For this review, take the finished solid that the model builds, in its own axes (mm). A direction names the side the tool comes from. Round coordinates to 2 decimals unless told otherwise and drop trailing zeros. Order: outer loops, then holes, each group sorted by start corner. A loop starts at its lowest first (then second) coordinate and runs counter-clockwise, first axis right, second up. Notation, with made-up numbers: (2.5, 55) - (40.5, 55) arc R16 ccw to (40.5, 60) - close; hole circle Ø7 at (65.5, -18.75). An arc over 180 degrees is marked (long way). One line per question, with ' | ' between items.
```python
from build123d import *

# Parameters (mm, degrees)
SKETCH1_W           = 5.75
SKETCH1_H           = 15.43
BOSS_EXTRUDE3_DEPTH = 11
SKETCH3_R           = 1
BOSS_EXTRUDE4_DEPTH = 3.086
SKETCH4_R           = 1
BOSS_EXTRUDE5_DEPTH = 1.543
BOSS_EXTRUDE6_START = -3.086
SKETCH5_R           = 1
BOSS_EXTRUDE6_DEPTH = 3.086


with BuildPart() as part:
    # Sketch1 → Boss-Extrude3 (new body)
    with BuildSketch(Plane(origin=(0, 0, 0), x_dir=(1, 0, 0), z_dir=(0, 1, 0))):
        with Locations((21.975, 0)):
            Rectangle(SKETCH1_W, SKETCH1_H)
    extrude(amount=BOSS_EXTRUDE3_DEPTH)

    # Sketch3 → Boss-Extrude4 (add)
    with BuildSketch(Plane(origin=(0, 0, -7.715), x_dir=(-1, 0, 0), z_dir=(0, 0, -1))):
        with BuildLine():
            Line((-24.85, 11), (-24.85, 6.250173181))
            Line((-24.85, 6.250173181), (-27.653680617, 6.250173181))
            ThreePointArc((-27.653680617, 6.250173181), (-29.999956704, 8.63934057), (-27.625, 11))
            Line((-27.625, 11), (-24.85, 11))
        make_face()
        with Locations((-27.625, 8.625)):
            Circle(SKETCH3_R, mode=Mode.SUBTRACT)
    extrude(amount=-BOSS_EXTRUDE4_DEPTH)

    # Sketch4 → Boss-Extrude5 (add, symmetric)
    with BuildSketch(Plane.XY):
        with BuildLine():
            Line((27.625, 11), (24.85, 11))
            Line((24.85, 11), (24.85, 6.250173181))
            Line((24.85, 6.250173181), (27.653680617, 6.250173181))
            ThreePointArc((27.653680617, 6.250173181), (29.999956704, 8.63934057), (27.625, 11))
        make_face()
        with Locations(Location((27.625, 8.625, 0), (0, 0, 180))):
            Circle(SKETCH4_R, mode=Mode.SUBTRACT)
    extrude(amount=BOSS_EXTRUDE5_DEPTH, both=True)

    # Sketch5 → Boss-Extrude6 (add)
    with BuildSketch(Plane.XY.offset(7.715).offset(BOSS_EXTRUDE6_START)):
        with BuildLine():
            Line((24.85, 6.250173181), (27.653680617, 6.250173181))
            ThreePointArc((27.653680617, 6.250173181), (29.999956704, 8.63934057), (27.625, 11))
            Line((27.625, 11), (24.85, 11))
            Line((24.85, 11), (24.85, 6.250173181))
        make_face()
        with Locations(Location((27.625, 8.625, 0), (0, 0, 180))):
            Circle(SKETCH5_R, mode=Mode.SUBTRACT)
    extrude(amount=BOSS_EXTRUDE6_DEPTH)


solid = part.part
```
(1) For probe 1 along Z at (x, y) = (25.25, 6.75) (3 decimals); probe 2 along X at (y, z) = (0.5, 4.75); probe 3 along Y at (x, z) = (25.5, 1.5), list the stretches that pass through material, from the lowest coordinate up. Write a range as [from, to].
Output values:
probe 1: [-7.715, -4.629], [-1.543, 1.543], [4.629, 7.715] | probe 2: [19.1, 24.85] | probe 3: [6.25, 11]
(2) We need section D-D on x = 29. State the section outline as (y, z) points (1 decimal), plus the area to 3 significant figures.
Output values:
outline: (6.7, -7.7) - (10.6, -7.7) - (10.6, -4.6) - (6.7, -4.6) - close; (6.7, -1.5) - (10.6, -1.5) - (10.6, 1.5) - (6.7, 1.5) - close; (6.7, 4.6) - (10.6, 4.6) - (10.6, 7.7) - (6.7, 7.7) - close | area: 35.9 mm^2
(3) For faces 5 (the flat face through (24.85, 4, 0)), 6 (the cylindrical face through (27.755, 7.634, -0.022)), 7 (the flat face through (26, 6.25, 6)), 8 (the flat face through (26, 9, 1.543)), list the 3-axis set-ups (+Z, -Z, +X, -X, +Y, -Y) from which the entire face can be reached by the end or side of a thin tool; tool diameter is ignored.
Output values:
face 5: +X, -Y | face 6: +Z, -Z | face 7: +Z, -Z, +X, -Y | face 8: +X, +Y, -Y
(4) We need section B-B on z = 5. State the section outline as (x, y) points (3 decimals), plus the area to 3 significant figures.
Output values:
outline: (19.1, 0) - (24.85, 0) - (24.85, 6.25) - (27.654, 6.25) arc R2.375 ccw to (27.625, 11) - (19.1, 11) - close; hole circle Ø2 at (27.625, 8.625) | area: 82.1 mm^2
(5) Insertion check: pin 1 (1.4 mm diameter, centred on x = 27, z = 6.5, fed in from -Y); pin 2 (1.5 mm diameter, centred on y = 7.5, z = -6, fed in from +X); pin 3 (1.5 mm diameter, centred on x = 27.5, y = 1.5, fed in from -Z) (3 decimals); pin 4 (4 mm diameter, centred on y = 5.5, z = 5.5, fed in from +X). Each pin has a flat end and moves straight along its axis. Give the tip position at first contact, or say it passes through.
Output values:
pin 1: y = 6.25 | pin 2: x = 29.97 | pin 3: through | pin 4: x = 29.72
(6) We need section A-A on x = 27.25. State the section outline as (y, z) points (3 decimals), plus the area to 3 significant figures.
Output values:
outline: (6.25, -7.715) - (7.698, -7.715) - (7.698, -4.629) - (6.25, -4.629) - close; (6.25, -1.543) - (7.698, -1.543) - (7.698, 1.543) - (6.25, 1.543) - close; (6.25, 4.629) - (7.698, 4.629) - (7.698, 7.715) - (6.25, 7.715) - close; (9.552, -7.715) - (11, -7.715) - (11, -4.629) - (9.552, -4.629) - close; (9.552, -1.543) - (11, -1.543) - (11, 1.543) - (9.552, 1.543) - close; (9.552, 4.629) - (11, 4.629) - (11, 7.715) - (9.552, 7.715) - close | area: 26.8 mm^2
(7) Mouldability with a two-part tool opening along Z and no side actions: class faces 1 (the flat face through (26, 9, -1.543)), 2 (the cylindrical face through (27.755, 9.616, -6.194)), 3 (the flat face through (23, 6, -7.715)), 4 (the flat face through (26, 9, 4.629)) as released by +Z, released by -Z, zero draft, split by the parting line, or undercut.
Output values:
face 1: undercut | face 2: zero draft | face 3: released by -Z | face 4: undercut
(8) We need section C-C on y = 9. State the section outline as (x, z) points (3 decimals), plus the area to 3 significant figures.
Output values:
outline: (19.1, -7.715) - (26.698, -7.715) - (26.698, -4.629) - (24.85, -4.629) - (24.85, -1.543) - (26.698, -1.543) - (26.698, 1.543) - (24.85, 1.543) - (24.85, 4.629) - (26.698, 4.629) - (26.698, 7.715) - (19.1, 7.715) - close; (28.552, -7.715) - (29.97, -7.715) - (29.97, -4.629) - (28.552, -4.629) - close; (28.552, -1.543) - (29.97, -1.543) - (29.97, 1.543) - (28.552, 1.543) - close; (28.552, 4.629) - (29.97, 4.629) - (29.97, 7.715) - (28.552, 7.715) - close | area: 119 mm^2
